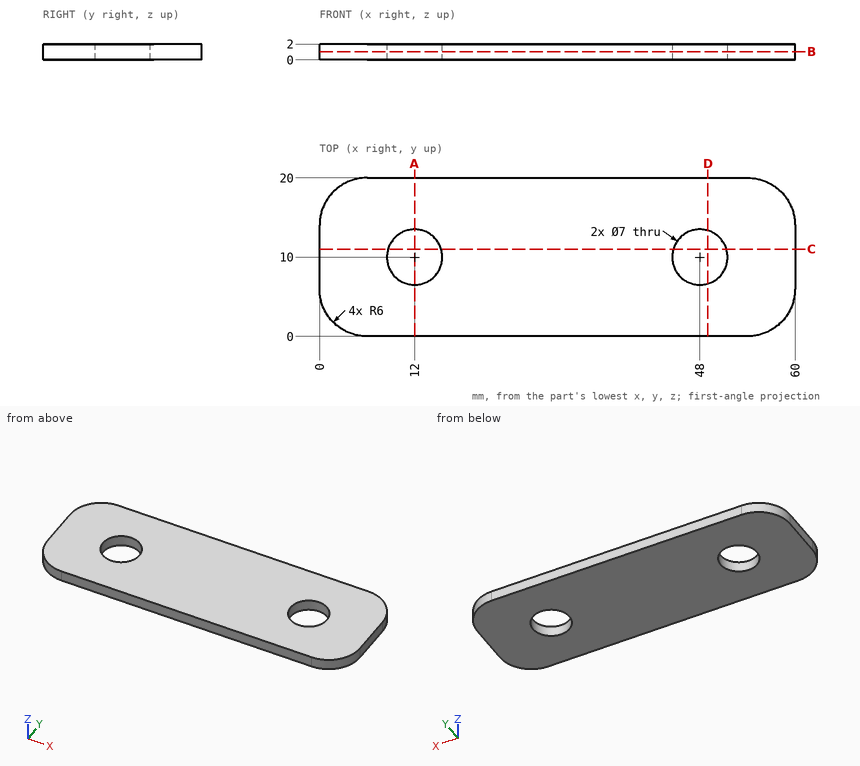
For this review, use the dimensioned drawing (mm, ordinates from the lowest corner) and the shaded views. Round coordinates to 2 decimals unless told otherwise and drop trailing zeros. Loops run counter-clockwise (first coordinate to the right, second up) from the corner with the lowest first, then second, coordinate; pieces in that order, holes last. Notation, with made-up numbers: M 27.25,37 L 75.25,37 A22 cw 75.25,69 Z; hole C 60,-22 d4. An arc over 180 degrees is marked long. Answer as a JSON object with one key per item and string values.
(1) Take a section at A-A on x = 12. Give the boundary of the cut face in (y, z), and give its area (3 significant figures).
Resolved:
{"outline": "M 0,0 L 6.5,0 L 6.5,2 L 0,2 Z; M 13.5,0 L 20,0 L 20,2 L 13.5,2 Z", "area": "26.0 mm²"}
(2) Take a section at C-C on y = 11. Give the boundary of the cut face in (x, z), and give its area (3 significant figures).
Resolved:
{"outline": "M 0,0 L 8.65,0 L 8.65,2 L 0,2 Z; M 15.35,0 L 44.65,0 L 44.65,2 L 15.35,2 Z; M 51.35,0 L 60,0 L 60,2 L 51.35,2 Z", "area": "93.2 mm²"}
(3) Clearance check with a flat-ended pin moving along its axis: P1, Ø5.5, axis at x = 12, y = 10, coming from the +Z side. State where the tip first meets the part, or that it passes through.
Resolved:
{"P1": "through"}
(4) To check wall thickness, follow line 1 along Y through (x, z) = (48, 0.85); line 2 along X through (y, z) = (13, 0.9); line 3 along X through (y, z) = (10.5, 1). State the ranges of each line that lie inside material, in increasing order.
Resolved:
{"line 1": "0 to 6.5, 13.5 to 20", "line 2": "0 to 10.2, 13.8 to 46.2, 49.8 to 60", "line 3": "0 to 8.54, 15.46 to 44.54, 51.46 to 60"}
(5) Take a section at D-D on x = 49. Give the boundary of the cut face in (y, z), and give its area (3 significant figures).
Resolved:
{"outline": "M 0,0 L 6.65,0 L 6.65,2 L 0,2 Z; M 13.35,0 L 20,0 L 20,2 L 13.35,2 Z", "area": "26.6 mm²"}
(6) Take a section at B-B on z = 1.05. Give the boundary of the cut face in (x, y), and give its area (3 significant figures).
Resolved:
{"outline": "M 0,6 A6 ccw 6,0 L 54,0 A6 ccw 60,6 L 60,14 A6 ccw 54,20 L 6,20 A6 ccw 0,14 Z; hole C 12,10 d7; hole C 48,10 d7", "area": "1,090 mm²"}
